```python
from build123d import *

# Parameters (mm, degrees)
SKETCH1_R           = 7.9375
BOSS_EXTRUDE1_DEPTH = 41.275
SKETCH4_OUTSIDE_W   = 34.984
SKETCH4_OUTSIDE_H   = 34.984
SKETCH4_OUTSIDE_R   = 6.35
CUT_EXTRUDE1_DEPTH  = 9.525
SKETCH5_OUTSIDE_W   = 34.984
SKETCH5_OUTSIDE_H   = 34.984
SKETCH5_OUTSIDE_R   = 6.35
CUT_EXTRUDE2_DEPTH  = 9.525
CUT_EXTRUDE3_DEPTH  = 63.5


with BuildPart() as part:
    # Sketch1 → Boss-Extrude1 (new body, symmetric)
    with BuildSketch(Plane(origin=(0, 0, 0), x_dir=(0, 0, -1), z_dir=(1, 0, 0))):
        Circle(SKETCH1_R)
    extrude(amount=BOSS_EXTRUDE1_DEPTH, both=True)

    # Sketch4 outside → Cut-Extrude1 (cut)
    with BuildSketch(Plane(origin=(41.275, 0, 0), x_dir=(0, 0, -1), z_dir=(1, 0, 0))):
        Rectangle(SKETCH4_OUTSIDE_W, SKETCH4_OUTSIDE_H)
        Circle(SKETCH4_OUTSIDE_R, mode=Mode.SUBTRACT)
    extrude(amount=-CUT_EXTRUDE1_DEPTH, mode=Mode.SUBTRACT)

    # Sketch5 outside → Cut-Extrude2 (cut)
    with BuildSketch(Plane.ZY.offset(41.275)):
        Rectangle(SKETCH5_OUTSIDE_W, SKETCH5_OUTSIDE_H)
        with Locations(Location((0, 0, 0), (0, 0, 180))):  # turned: the seam where the file's is
            Circle(SKETCH5_OUTSIDE_R, mode=Mode.SUBTRACT)
    extrude(amount=-CUT_EXTRUDE2_DEPTH, mode=Mode.SUBTRACT)

    # Sketch7 → Cut-Extrude3 (cut)
    with BuildSketch(Plane.ZY.offset(31.75)):
        with BuildLine():
            Line((0, 5.55625), (2.38125, 5.55625))
            Line((2.38125, 5.55625), (2.38125, 7.571892411))
            ThreePointArc((2.38125, 7.571892411), (0, 7.9375), (-2.38125, 7.571892411))
            Line((-2.38125, 7.571892411), (-2.38125, 5.55625))
            Line((-2.38125, 5.55625), (0, 5.55625))
        make_face()
    extrude(amount=-CUT_EXTRUDE3_DEPTH, mode=Mode.SUBTRACT)


solid = part.part
```
Source: CAD feature listing. Evaluate the final solid. Frame: model axes, mm. A direction names the side the tool comes from. Coordinates: 2 decimals unless noted, no trailing zeros. Loops run counter-clockwise (first coordinate to the right, second up) from the corner with the lowest first, then second, coordinate; pieces in that order, holes last. Notation, with made-up numbers: M 87.5,-23.75 L 116.5,-23.75 A27 cw 116.5,-7.75 Z; hole C 44,2 d11. An arc over 180 degrees is marked long. Use a Markdown table: item, result. Add a question column.
Q1. Material intervals for L1, parallel to X at y = 3.75, z = -6.75; L2, parallel to Y at x = 6.5, z = 4.75; L3, parallel to Y at x = -12.5, z = -0.5, sorted ascending.
Q2. Section query C-C, the plane x = -16.5. Return loops of the section in (y, z) (1 decimal).
Q3. Access query for faces 1 (the flat face through (-41.275, 0, 0)), 2 (the cylindrical face through (36.58, -6.2, 1.38)), 3 (the flat face through (0, 5.556, 0)), 4 (the flat face through (-31.75, -6.5, 0.6)). Directions: +Z, -Z, +X, -X, +Y, -Y. A direction counts if a zero-diameter tool reaches every point of the face in a straight line with its end or side. Return the directions, or none.
Q4. First-contact query: pin 1 (1.6 mm diameter, centred on x = 11.5, y = 6, fed in from -Z); pin 2 (1 mm diameter, centred on x = 8, y = 6.5, fed in from +Z); pin 3 (2 mm diameter, centred on x = -28.5, y = -1.5, fed in from +Z). Flat tips, straight axial feed; report the tip coordinate or a pass-through.
Q5. Draft query along X for faces 5 (the flat face through (0, 7, 2.381)), 6 (the cylindrical face through (-36.579, 5.634, -2.93)), 7 (the flat face through (41.275, 0, 0)). Return one class per face: pulls with the +X half, pulls with the -X half, needs draft (parallel to the pull), parting line crosses it, or undercut.
Q6. Section query D-D, the plane x = -34.5. Return loops of the section in (y, z).
Result:
| question | item | result |
|---|---|---|
| 1 | L1 | x = -31.75 to 31.75 |
| 1 | L2 | y = -6.36 to 6.36 |
| 1 | L3 | y = -7.92 to 5.56 |
| 2 | outline | M 5.6,-2.4 L 5.6,2.4 L 7.6,2.4 A7.9 ccw long 7.6,-2.4 Z |
| 3 | face 1 | +Z, -Z, -X, +Y, -Y |
| 3 | face 2 | +X |
| 3 | face 3 | +Y |
| 3 | face 4 | -X |
| 4 | pin 1 | stops at z = -6 |
| 4 | pin 2 | stops at z = 5.2 |
| 4 | pin 3 | stops at z = 7.92 |
| 5 | face 5 | undercut |
| 5 | face 6 | needs draft |
| 5 | face 7 | pulls with the +X half |
| 6 | outline | C 0,0 d12.7 |
